Geometry: final body of the model. Coordinates: model frame, mm. A direction names the side the tool comes from. Coordinates: 2 decimals unless noted, no trailing zeros. Order: outer loops, then holes, each group sorted by start corner. A loop starts at its lowest first (then second) coordinate and runs counter-clockwise, first axis right, second up. Notation, with made-up numbers: (33, 71.5) -> (47, 71.5) arc R20 cw to (47, 84.5) -> close; hole circle Ø2 at (-2, -9.5). An arc over 180 degrees is marked (long way). Answer in a Markdown table with one row per item. Add a question column.
1) Section query D-D on y = 20.5. Return the cut outline in (x, z).
2) Ray query, line 1 (X direction, y = 6, z = 39) (3 decimals); line 2 (Z direction, x = 0, y = 14). Return the intervals inside material, ascending. Write a range as from..to.
3) Section query B-B on z = 69.85. Return the cut outline in (x, y) (3 decimals), then the cut area to 3 significant figures.
4) Contact query for flat-ended pins moving along their axis: P1, Ø1.5, axis at x = 39.5, y = -8, coming from the -Z side; P2, Ø20.5, axis at x = -2.5, z = 25.5, coming from the -Y side (3 decimals); P3, Ø10, axis at x = 0, z = 69.85, coming from the +Y side (3 decimals); P4, Ø7.5, axis at y = -1.5, z = 39.5, coming from the -X side (3 decimals). Output: stop coordinate, or through.
5) Set-up query: faces 1 (the face through (0, 12.7, 44)), 2 (the face through (15.875, 0, 44)), 3 (the face through (0, -15.875, 44)). Return all of +Z, -Z, +X, -X, +Y, -Y with unobstructed straight access to the full face (end or side cutting, diameter ignored); none if empty.
6) Pull-direction query (X, two-part tool) for faces 4 (the face through (50.8, -1, 3)), 5 (the face through (-1, -50.8, 3)), 6 (the face through (-0.83, 14.27, 66.13)); classes: +X half, -X half, draft (parallel to the pull), parting line (faces both ways), or undercut.
7) Section query A-A on x = 0. Return the cut outline in (y, z) (3 decimals), then the cut area to 3 significant figures.
8) Section query C-C on z = 46. Return the cut outline in (x, y) (3 decimals).
```python
from build123d import *

# Parameters (mm, degrees)
F0_W     = 101.6
F0_H     = 101.6
F1_DEPTH = 6.35
F2_W     = 31.75
F2_H     = 31.75
F2_W_2   = 25.4
F2_H_2   = 25.4
F3_DEPTH = 76.2
F4_R     = 3.81
F5_DEPTH = 66.676


with BuildPart() as f1:
    # F0 (on Top) → F1 (new body)
    with BuildSketch(Plane.XY):
        Rectangle(F0_W, F0_H)
    extrude(amount=F1_DEPTH)

    # F2 (on face) → F3 (join)
    with BuildSketch(Plane.XY.offset(6.35)):
        Rectangle(F2_W, F2_H)
        Rectangle(F2_W_2, F2_H_2, mode=Mode.SUBTRACT)
    extrude(amount=F3_DEPTH)

    # F4 (on face) → F5 (cut, through all)
    with BuildSketch(Plane.XZ.offset(15.875)):
        with Locations((0, 69.85)):
            Circle(F4_R)
    extrude(amount=-F5_DEPTH, mode=Mode.SUBTRACT)


solid = f1.part
```
Result:
| question | item | result |
|---|---|---|
| 1 | outline | (-50.8, 0) -> (50.8, 0) -> (50.8, 6.35) -> (-50.8, 6.35) -> close |
| 2 | line 1 | -15.875..-12.7, 12.7..15.875 |
| 2 | line 2 | 0..66.04, 73.66..82.55 |
| 3 | outline | (-15.875, -15.875) -> (-3.81, -15.875) -> (-3.81, -12.7) -> (-12.7, -12.7) -> (-12.7, 12.7) -> (-3.81, 12.7) -> (-3.81, 15.875) -> (-15.875, 15.875) -> close; (3.81, -15.875) -> (15.875, -15.875) -> (15.875, 15.875) -> (3.81, 15.875) -> (3.81, 12.7) -> (12.7, 12.7) -> (12.7, -12.7) -> (3.81, -12.7) -> close |
| 3 | area | 315 mm2 |
| 4 | P1 | z = 0 |
| 4 | P2 | y = -15.875 |
| 4 | P3 | y = 15.875 |
| 4 | P4 | x = -15.875 |
| 5 | face 1 | +Z |
| 5 | face 2 | +Z, +X, +Y, -Y |
| 5 | face 3 | +Z, +X, -X, -Y |
| 6 | face 4 | +X half |
| 6 | face 5 | draft |
| 6 | face 6 | undercut |
| 7 | outline | (-50.8, 0) -> (50.8, 0) -> (50.8, 6.35) -> (15.875, 6.35) -> (15.875, 66.04) -> (12.7, 66.04) -> (12.7, 6.35) -> (-12.7, 6.35) -> (-12.7, 66.04) -> (-15.875, 66.04) -> (-15.875, 6.35) -> (-50.8, 6.35) -> close; (-15.875, 73.66) -> (-12.7, 73.66) -> (-12.7, 82.55) -> (-15.875, 82.55) -> close; (12.7, 73.66) -> (15.875, 73.66) -> (15.875, 82.55) -> (12.7, 82.55) -> close |
| 7 | area | 1,080 mm2 |
| 8 | outline | (-15.875, -15.875) -> (15.875, -15.875) -> (15.875, 15.875) -> (-15.875, 15.875) -> close; hole (-12.7, -12.7) -> (12.7, -12.7) -> (12.7, 12.7) -> (-12.7, 12.7) -> close |
